Build history of the part. All positions in model axes, mm. Round coordinates to 2 decimals unless told otherwise and drop trailing zeros. Write each loop counter-clockwise with the first axis right and the second up, starting at its lowest first coordinate (ties: lowest second). Pieces come first, ordered by that corner, then holes. Notation, with made-up numbers: M -3.75,-15 L 28.25,-15 A21 ccw 28.25,0 Z; hole C 80.5,73 d11. An arc over 180 degrees is marked long. Write item = value, one per line. Start each with the question number.
Q1. Band-saw the part on B-B on x = 0.5. Write the cut outline in (y, z).
Q2. Probe L1, parallel to Z at x = 5, y = 6; L2, parallel to X at y = 2.75, z = 22; L3, parallel to Z at x = 3.5, y = 5.5. List the from-to ranges inside material, lowest first.
Q3. Band-saw the part on A-A on x = 3.5. Write the cut outline in (y, z), plus the area to 3 significant figures.
Q4. Pull direction X, two halves, no side cores. Call faces 1 (the flat face through (0, 3, 9)), 2 (the cylindrical face through (3, 3.9, 20)), 3 (the flat face through (7, 3, 9)): released by +X, released by -X, zero draft, split by the parting line, or undercut.
Q5. Band-saw the part on C-C on x = 5. Write the cut outline in (y, z).
Q6. Drop flat-ended pins along their axis: P1, Ø4, axis at x = 3, y = 6, coming from the +Z side; P2, Ø2, axis at x = 5, y = 2.5, coming from the +Z side. Give the stop position or say it passes through.
```python
from build123d import *

# Parameters (mm, degrees)
SKETCH1_W           = 7
SKETCH1_H           = 7
BOSS_EXTRUDE1_DEPTH = 20
BOSS_EXTRUDE2_DEPTH = 7
SKETCH5_W           = 7
SKETCH5_H           = 7
BOSS_EXTRUDE4_DEPTH = 10
SKETCH4_R           = 2.25
CUT_EXTRUDE1_DEPTH  = 27.162950904


with BuildPart() as part:
    # Sketch1 → Boss-Extrude1 (new body)
    with BuildSketch(Plane.XY):
        with Locations((3.5, 3.5)):
            Rectangle(SKETCH1_W, SKETCH1_H)
    extrude(amount=BOSS_EXTRUDE1_DEPTH)

    # Sketch3 → Boss-Extrude2 (add)
    with BuildSketch(Plane(origin=(7, 0, 0), x_dir=(0, 0, -1), z_dir=(1, 0, 0))):
        Polygon((-20, 7), (-27, 7), (-20, 0), align=None)
    extrude(amount=-BOSS_EXTRUDE2_DEPTH)

    # Sketch5 → Boss-Extrude4 (add)
    with BuildSketch(Plane(origin=(0, 0, 0), x_dir=(-1, 0, 0), z_dir=(0, 0, -1))):
        with Locations((-3.5, 3.5)):
            Rectangle(SKETCH5_W, SKETCH5_H)
    extrude(amount=BOSS_EXTRUDE4_DEPTH)

    # Sketch4 → Cut-Extrude1 (cut, through all)
    with BuildSketch(Plane(origin=(0, -10, 10), x_dir=(1, 0, 0), z_dir=(0, -0.707106781, 0.707106781))):
        with Locations((3.5, 19.091883092)):
            Circle(SKETCH4_R)
    extrude(amount=-CUT_EXTRUDE1_DEPTH, mode=Mode.SUBTRACT)


solid = part.part
```
Conclusion:
q1.outline = M 0,-10 L 7,-10 L 7,27 L 0,20 Z
q2.L1 = -10 to 18.63, 23.37 to 26
q2.L2 = 0 to 1.91, 5.09 to 7
q2.L3 = -10 to 18.32, 24.68 to 25.5
q3.outline = M 0,-10 L 7,-10 L 7,16.82 L 1.91,21.91 L 0,20 Z; M 5.09,25.09 L 7,23.18 L 7,27 Z
q3.area = 212 mm^2
q4.face_1 = released by -X
q4.face_2 = undercut
q4.face_3 = released by +X
q5.outline = M 0,-10 L 7,-10 L 7,17.63 L 2.31,22.31 L 0,20 Z; M 4.69,24.69 L 7,22.37 L 7,27 Z
q6.P1 = 27
q6.P2 = 23.2
